The listing builds one solid part. Answer for the finished solid, in the listing's coordinates (mm). Face numbers are marked on the shaded views. Round coordinates to 2 decimals unless told otherwise and drop trailing zeros. Answer in a Markdown table with one row per item.
from build123d import *

# Parameters (mm, degrees)
BOSS_EXTRUDE1_DEPTH = 6.35
SKETCH2_R           = 1.5875
CUT_EXTRUDE1_DEPTH  = 38.1
CUT_EXTRUDE2_DEPTH  = 6.35
LPATTERN1_COUNT     = 11
LPATTERN1_PITCH     = 2.54
CUT_EXTRUDE3_START  = -6.35
CUT_EXTRUDE3_DEPTH  = 6.35
CIRPATTERN1_COUNT   = 3
CIRPATTERN1_ANGLE   = 68
BOSS_EXTRUDE2_DEPTH = 6.35
BOSS_EXTRUDE3_START = 0.508
BOSS_EXTRUDE3_DEPTH = 0.508
FILLET3_R           = 0.762


with BuildPart() as part:
    # Sketch1 → Boss-Extrude1 (new body)
    with BuildSketch(Plane(origin=(0, 0, 0), x_dir=(0, 0, -1), z_dir=(1, 0, 0))):
        with BuildLine():
            Line((0, -4.7625), (12.7, -4.7625))
            ThreePointArc((12.7, -4.7625), (16.69058737, -2.599349668), (17.05608691, 1.925074826))
            Line((17.05608691, 1.925074826), (3.957741706, 31.564198098))
            ThreePointArc((3.957741706, 31.564198098), (-1.413387908, 34.29219694), (-5.160415138, 29.575121793))
            Line((-5.160415138, 29.575121793), (-4.762069934, -0.064001479))
            ThreePointArc((-4.762069934, -0.064001479), (-3.344891568, -3.39014847), (0, -4.7625))
        make_face()
    extrude(amount=BOSS_EXTRUDE1_DEPTH)

    # Sketch2 → Cut-Extrude1 (cut)
    with BuildSketch(Plane(origin=(6.35, 0, 0), x_dir=(0, 0, -1), z_dir=(1, 0, 0))):
        Circle(SKETCH2_R)
        with Locations((12.7, 0)):
            Circle(SKETCH2_R)
    extrude(amount=-CUT_EXTRUDE1_DEPTH, mode=Mode.SUBTRACT)

    # Sketch3 → Cut-Extrude2 (cut)
    with BuildSketch(Plane(origin=(6.35, 0, 0), x_dir=(0, 0, -1), z_dir=(1, 0, 0))):
        Polygon((-4.782550408, 1.4598609), (-4.792790644, 2.22179209), (-4.035979573, 2.612997921), (-4.0154991, 1.089135542), align=None)
    cut_extrude2 = extrude(amount=-CUT_EXTRUDE2_DEPTH, mode=Mode.SUBTRACT)

    # LPattern1: Cut-Extrude2 ×11
    with Locations(*[Vector(0, 0.9999096975250266, 0.013438630711869543) * (i * LPATTERN1_PITCH) for i in range(1, LPATTERN1_COUNT)]):
        add(cut_extrude2, mode=Mode.SUBTRACT)

    # Sketch5 → Cut-Extrude3 (cut)
    with BuildSketch(Plane(origin=(6.35, 0, 0), x_dir=(0, 0, -1), z_dir=(1, 0, 0)).offset(CUT_EXTRUDE3_START)):
        with BuildLine():
            Line((-2.14250095, 34.070751301), (-2.285611832, 33.230915438))
            Line((-2.285611832, 33.230915438), (-0.827385747, 33.673806717))
            Line((-0.827385747, 33.673806717), (-1.413387908, 34.29219694))
            ThreePointArc((-1.413387908, 34.29219694), (-1.782380451, 34.196079788), (-2.14250095, 34.070751301))
        make_face()
    cut_extrude3 = extrude(amount=CUT_EXTRUDE3_DEPTH, mode=Mode.SUBTRACT)

    # CirPattern1: Cut-Extrude3 ×3 about axis
    cirpattern1_axis = Axis((0, 29.639123272, 0.398345204), (1, 0, 0))
    for i in range(1, CIRPATTERN1_COUNT):
        add(cut_extrude3.rotate(cirpattern1_axis, i * CIRPATTERN1_ANGLE / (CIRPATTERN1_COUNT - 1)), mode=Mode.SUBTRACT)

    # Sketch6 → Boss-Extrude2 (add)
    with BuildSketch(Plane(origin=(0, 0, 0), x_dir=(0, 0, -1), z_dir=(1, 0, 0))):
        with BuildLine():
            Line((-7.335974688, 2.441635031), (-7.70018577, 29.540987671))
            ThreePointArc((-7.70018577, 29.540987671), (-7.343715671, 31.89485715), (-6.249061464, 34.008977446))
            ThreePointArc((-6.249061464, 34.008977446), (-3.897096462, 35.275278165), (-1.413387908, 34.29219694))
            ThreePointArc((-1.413387908, 34.29219694), (-1.118769293, 34.346818609), (-0.821298902, 34.382805009))
            ThreePointArc((-0.821298902, 34.382805009), (-3.75592559, 35.788432355), (-6.656067812, 34.312967301))
            ThreePointArc((-6.656067812, 34.312967301), (-7.826871877, 32.051777768), (-8.208139896, 29.534160847))
            Line((-8.208139896, 29.534160847), (-7.844020566, 2.441635031))
            ThreePointArc((-7.844020566, 2.441635031), (-6.92684089, 0.288995326), (-4.762069934, -0.599172997))
            Line((-4.762069934, -0.599172997), (-4.724658503, -0.599172997))
            ThreePointArc((-4.724658503, -0.599172997), (-4.750905835, -0.332114438), (-4.762069934, -0.064001479))
            ThreePointArc((-4.762069934, -0.064001479), (-6.567956624, 0.655743647), (-7.335974688, 2.441635031))
        make_face()
    extrude(amount=BOSS_EXTRUDE2_DEPTH)

    # Sketch7 → Boss-Extrude3 (add)
    with BuildSketch(Plane.ZY.offset(BOSS_EXTRUDE3_START)):
        with BuildLine():
            Line((3.890529822, 29.592188854), (3.484762618, -0.599172997))
            Line((3.484762618, -0.599172997), (4.762069934, -0.599172997))
            ThreePointArc((4.762069934, -0.599172997), (6.92684089, 0.288995326), (7.844020566, 2.441635031))
            Line((7.844020566, 2.441635031), (8.208139896, 29.534160847))
            ThreePointArc((8.208139896, 29.534160847), (7.826871877, 32.051777768), (6.656067812, 34.312967301))
            ThreePointArc((6.656067812, 34.312967301), (3.75592559, 35.788432355), (0.821298902, 34.382805009))
            Line((0.821298902, 34.382805009), (-0.201439925, 33.079735725))
            ThreePointArc((-0.201439925, 33.079735725), (2.663789861, 32.297189628), (3.890529822, 29.592188854))
        make_face()
    extrude(amount=-BOSS_EXTRUDE3_DEPTH)

    # Fillet3
    fillet3_edges = [part.edges().sort_by_distance(p)[0] for p in [
        (6.35, -2.599349668, -16.69058737),
        (6.35, 16.744636462, -10.506914308),
        (6.35, 33.741303888, -2.021059773),
        (0, -3.573161601, 3.148638186),
        (6.35, -3.573161601, 3.148638186),
        (0, 33.741303888, -2.021059773),
        (0, 16.744636462, -10.506914308),
        (6.35, -4.7625, -6.35),
        (0, -2.599349668, -16.69058737),
        (0, -4.7625, -6.35),
    ]]
    fillet(fillet3_edges, radius=FILLET3_R)


solid = part.part
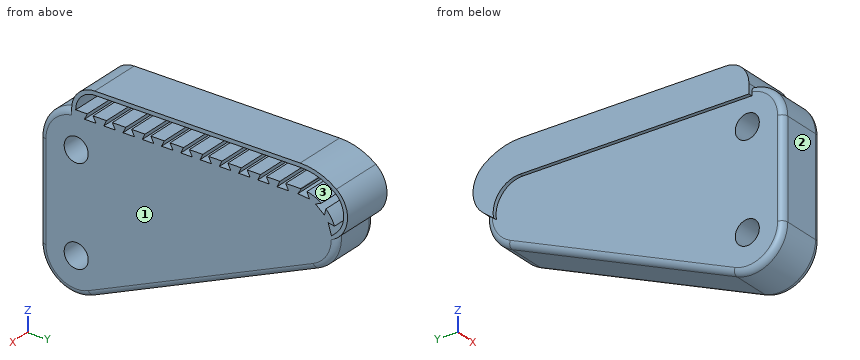
(1) Find the intervals of material crossed by line 1 (Z direction, x = 0.75, y = -1); line 2 (Y direction, x = 3.5, z = -12.5); line 3 (X direction, y = 31.5, z = 6.25), in increasing order.
Checked values:
| item | result |
|---|---|
| line 1 | z = -17.36 to -13.93, -11.47 to -1.23, 1.23 to 4.66 |
| line 2 | y = -4.76 to -1.57, 1.57 to 12.23 |
| line 3 | x = -0.51 to 0 |
(2) Flat-ended cylindrical pins translate along their axes: pin 1 (1 mm diameter, centred on x = 3, y = 17, fed in from +Z); pin 2 (3.5 mm diameter, centred on y = 0, z = -12.7, fed in from -X); pin 3 (1.4 mm diameter, centred on x = 4, z = 4.5, fed in from -Y). Find the tip coordinate at first contact, or state that the pin passes through.
Checked values:
| item | result |
|---|---|
| pin 1 | stops at z = 8.05 |
| pin 2 | stops at x = 0 |
| pin 3 | stops at y = -2.87 |
(3) For a pull along Y with two mould halves and no side action, classify the marked faces 1, 2 and 3 as pulls with the +Y half, pulls with the -Y half, needs draft (parallel to the pull), parting line crosses it, or undercut.
Checked values:
| item | result |
|---|---|
| face 1 | needs draft |
| face 2 | pulls with the -Y half |
| face 3 | undercut |
(4) Section A-A (x = 3) is taken. State how many separate pieces and enclosed holes the cut face has, and give its area (3 significant figures).
Checked values:
| item | result |
|---|---|
| separate pieces | 1 |
| enclosed holes | 3 |
| area | 609 mm2 |
